Work out the finished part from the listing and answer in its coordinate system (mm). Coordinates: 2 decimals unless noted, no trailing zeros. Use CSV: the item, a comma, the result in double quotes. Start each with the question number.
from build123d import *

# Parameters (mm, degrees)
SKETCH_2_W          = 9
SKETCH_2_H          = 6.5
EXTRUDE_1_DEPTH     = 410
SKETCH_3_R          = 3
CUT_EXTRUDE_1_DEPTH = 3.5
SKETCH_4_R          = 1.75
CUT_EXTRUDE_2_DEPTH = 411.076212429


with BuildPart() as part:
    # 草图2 → 凸台-拉伸1 (new body)
    with BuildSketch(Plane(origin=(0, 0, 0), x_dir=(0, 0, -1), z_dir=(1, 0, 0))):
        Rectangle(SKETCH_2_W, SKETCH_2_H)
    extrude(amount=EXTRUDE_1_DEPTH)

    # 草图3 → 切除-拉伸1 (cut)
    with BuildSketch(Plane(origin=(0, 3.25, 0), x_dir=(1, 0, 0), z_dir=(0, 1, 0))):
        with Locations(Location((15, 0, 0), (0, 0, 270))):
            Circle(SKETCH_3_R)
        with Locations(Location((35, 0, 0), (0, 0, 270))):
            Circle(SKETCH_3_R)
        with Locations(Location((55, 0, 0), (0, 0, 270))):
            Circle(SKETCH_3_R)
        with Locations(Location((75, 0, 0), (0, 0, 270))):
            Circle(SKETCH_3_R)
        with Locations(Location((95, 0, 0), (0, 0, 270))):
            Circle(SKETCH_3_R)
        with Locations(Location((115, 0, 0), (0, 0, 270))):
            Circle(SKETCH_3_R)
        with Locations(Location((135, 0, 0), (0, 0, 270))):
            Circle(SKETCH_3_R)
        with Locations(Location((155, 0, 0), (0, 0, 270))):
            Circle(SKETCH_3_R)
        with Locations(Location((175, 0, 0), (0, 0, 270))):
            Circle(SKETCH_3_R)
        with Locations(Location((195, 0, 0), (0, 0, 270))):
            Circle(SKETCH_3_R)
        with Locations(Location((215, 0, 0), (0, 0, 270))):
            Circle(SKETCH_3_R)
        with Locations(Location((235, 0, 0), (0, 0, 270))):
            Circle(SKETCH_3_R)
        with Locations(Location((255, 0, 0), (0, 0, 270))):
            Circle(SKETCH_3_R)
        with Locations(Location((275, 0, 0), (0, 0, 270))):
            Circle(SKETCH_3_R)
        with Locations(Location((295, 0, 0), (0, 0, 270))):
            Circle(SKETCH_3_R)
        with Locations(Location((315, 0, 0), (0, 0, 270))):
            Circle(SKETCH_3_R)
        with Locations(Location((335, 0, 0), (0, 0, 270))):
            Circle(SKETCH_3_R)
        with Locations(Location((355, 0, 0), (0, 0, 270))):
            Circle(SKETCH_3_R)
        with Locations(Location((375, 0, 0), (0, 0, 270))):
            Circle(SKETCH_3_R)
        with Locations(Location((395, 0, 0), (0, 0, 270))):
            Circle(SKETCH_3_R)
    extrude(amount=-CUT_EXTRUDE_1_DEPTH, mode=Mode.SUBTRACT)

    # 草图4 → 切除-拉伸2 (cut, through all)
    with BuildSketch(Plane(origin=(0, 3.25, 0), x_dir=(1, 0, 0), z_dir=(0, 1, 0))):
        with Locations(Location((15, 0, 0), (0, 0, 270))):
            Circle(SKETCH_4_R)
        with Locations(Location((35, 0, 0), (0, 0, 270))):
            Circle(SKETCH_4_R)
        with Locations(Location((55, 0, 0), (0, 0, 270))):
            Circle(SKETCH_4_R)
        with Locations(Location((75, 0, 0), (0, 0, 270))):
            Circle(SKETCH_4_R)
        with Locations(Location((95, 0, 0), (0, 0, 270))):
            Circle(SKETCH_4_R)
        with Locations(Location((115, 0, 0), (0, 0, 270))):
            Circle(SKETCH_4_R)
        with Locations(Location((135, 0, 0), (0, 0, 270))):
            Circle(SKETCH_4_R)
        with Locations(Location((155, 0, 0), (0, 0, 270))):
            Circle(SKETCH_4_R)
        with Locations(Location((175, 0, 0), (0, 0, 270))):
            Circle(SKETCH_4_R)
        with Locations(Location((195, 0, 0), (0, 0, 270))):
            Circle(SKETCH_4_R)
        with Locations(Location((215, 0, 0), (0, 0, 270))):
            Circle(SKETCH_4_R)
        with Locations(Location((235, 0, 0), (0, 0, 270))):
            Circle(SKETCH_4_R)
        with Locations(Location((255, 0, 0), (0, 0, 270))):
            Circle(SKETCH_4_R)
        with Locations(Location((275, 0, 0), (0, 0, 270))):
            Circle(SKETCH_4_R)
        with Locations(Location((295, 0, 0), (0, 0, 270))):
            Circle(SKETCH_4_R)
        with Locations(Location((315, 0, 0), (0, 0, 270))):
            Circle(SKETCH_4_R)
        with Locations(Location((335, 0, 0), (0, 0, 270))):
            Circle(SKETCH_4_R)
        with Locations(Location((355, 0, 0), (0, 0, 270))):
            Circle(SKETCH_4_R)
        with Locations(Location((375, 0, 0), (0, 0, 270))):
            Circle(SKETCH_4_R)
        with Locations(Location((395, 0, 0), (0, 0, 270))):
            Circle(SKETCH_4_R)
    extrude(amount=-CUT_EXTRUDE_2_DEPTH, mode=Mode.SUBTRACT)


solid = part.part
Item 1: A cutting plane is placed at A-A (y = -2.25). Count the separate pieces of the cut face and the enclosed holes in it, then the cut area to 3 significant figures.
Item 2: Straight lines are drawn through the part: probe 1 along Z at (x, y) = (275, 1.45); probe 2 along Z at (x, y) = (195, -1.3); probe 3 along Y at (x, z) = (74, 2.75). For each, find the intervals that lie inside material, in ascending order. Write a range as [from, to].
Item 3: This flat-tipped pin is pushed along its axis until it touches: pin 1 (1.8 mm diameter, centred on x = 195.5, z = 0, fed in from +Y). Where does it stop, or does it pass through?
Calculated:
1,separate pieces,"1"
1,enclosed holes,"20"
1,area,"3,500 mm²"
2,probe 1,"z = [-4.5, -3], [3, 4.5]"
2,probe 2,"z = [-4.5, -1.75], [1.75, 4.5]"
2,probe 3,"y = [-3.25, -0.25]"
3,pin 1,"passes through"
